Here's how the part is built. I have some questions about the finished solid (model axes, mm). A direction names the side the tool comes from. Round coordinates to 2 decimals unless told otherwise and drop trailing zeros. Order: outer loops, then holes, each group sorted by start corner. A loop starts at its lowest first (then second) coordinate and runs counter-clockwise, first axis right, second up. Notation, with made-up numbers: (-38, 80) -> (8, 80) arc R24 cw to (8, 92) -> close; hole circle Ø6 at (-5.5, 81). An arc over 180 degrees is marked (long way). One line per item, written item: value.
```python
from build123d import *
from build123d.topology import SkipClean

# Parameters (mm, degrees)
SKETCH_2_R          = 4.9
EXTRUDE_1_DEPTH     = 9
EXTRUDE_2_DEPTH     = 10
SKETCH_4_R          = 1.5
CUT_EXTRUDE_1_DEPTH = 22.46392322
SKETCH_5_R          = 3.35
EXTRUDE_3_DEPTH     = 34
CHAMFER_1_SIZE      = 1


with BuildPart() as part:
    # 草图2 → 凸台-拉伸1 (new body)
    with BuildSketch(Plane.XY):
        Circle(SKETCH_2_R)
    extrude(amount=EXTRUDE_1_DEPTH)

    # 草图3 → 凸台-拉伸2 (add)
    with SkipClean():  # the faces are left unmerged after this step: merging them gives an invalid solid
        with BuildSketch(Plane.XY.offset(9)):
            with BuildLine():
                Line((-1.8, -4.557411546), (-1.8, 4.557411546))
                ThreePointArc((-1.8, 4.557411546), (-2.894085134, 3.954019631), (-3.8, 3.09354166))
                Line((-3.8, 3.09354166), (-3.8, -3.09354166))
                ThreePointArc((-3.8, -3.09354166), (-2.894085134, -3.954019631), (-1.8, -4.557411546))
            make_face()
            with BuildLine():
                Line((1.8, -4.557411546), (1.8, 4.557411546))
                ThreePointArc((1.8, 4.557411546), (2.894085134, 3.954019631), (3.8, 3.09354166))
                Line((3.8, 3.09354166), (3.8, -3.09354166))
                ThreePointArc((3.8, -3.09354166), (2.894085134, -3.954019631), (1.8, -4.557411546))
            make_face()
        extrude(amount=EXTRUDE_2_DEPTH)

    # 草图4 → 切除-拉伸1 (cut, through all)
    with SkipClean():  # the faces are left unmerged after this step: merging them gives an invalid solid
        with BuildSketch(Plane.ZY.offset(3.8)):
            with Locations((16.318814586, 0)):
                Circle(SKETCH_4_R)
        extrude(amount=-CUT_EXTRUDE_1_DEPTH, mode=Mode.SUBTRACT)

    # 草图5 → 凸台-拉伸3 (add)
    with SkipClean():  # the faces are left unmerged after this step: merging them gives an invalid solid
        with BuildSketch(Plane(origin=(0, 0, 0), x_dir=(-1, 0, 0), z_dir=(0, 0, -1))):
            with Locations(Location((0, 0, 0), (0, 0, 180))):
                Circle(SKETCH_5_R)
        extrude(amount=EXTRUDE_3_DEPTH)

    # 倒角1
    chamfer_1_edges = [part.edges().sort_by_distance(p)[0] for p in [
        (-3.35, 0, -34),
    ]]
    chamfer(chamfer_1_edges, length=CHAMFER_1_SIZE)


solid = part.part
```
Q1. I want a section at A-A on z = 13. Write out the boundary of the cut face in (x, y), then the cut area to 3 significant figures.
Answers:
outline: (-3.8, -3.09) arc R4.9 ccw to (-1.8, -4.56) -> (-1.8, 4.56) arc R4.9 ccw to (-3.8, 3.09) -> close; (1.8, -4.56) arc R4.9 ccw to (3.8, -3.09) -> (3.8, 3.09) arc R4.9 ccw to (1.8, 4.56) -> close
area: 31.7 mm2
Q2. I want a section at B-B on x = 0. Write out the boundary of the cut face in (y, z), then the cut area to 3 significant figures.
Answers:
outline: (-4.9, 0) -> (-3.35, 0) -> (-3.35, -33) -> (-2.35, -34) -> (2.35, -34) -> (3.35, -33) -> (3.35, 0) -> (4.9, 0) -> (4.9, 9) -> (-4.9, 9) -> close
area: 315 mm2
Q3. Which directions (+Z, -Z, +X, -X, +Y, -Y) give clear straight access to the entire face, cutting with the end or side of a thin tool? Please do faces 5 (the face through (-4, 0, 9)), 6 (the face through (-3, 0, 19)), 7 (the face through (0, 0, 9)), 8 (the face through (4, 0, 9)).
Answers:
face 5: +Z, -X, +Y, -Y
face 6: +Z, +X, -X, +Y, -Y
face 7: +Z, +Y, -Y
face 8: +Z, +X, +Y, -Y
Q4. I want a section at C-C on y = 0. Write out the boundary of the cut face in (x, z).
Answers:
outline: (-4.9, 0) -> (-3.35, 0) -> (-3.35, -33) -> (-2.35, -34) -> (2.35, -34) -> (3.35, -33) -> (3.35, 0) -> (4.9, 0) -> (4.9, 9) -> (3.8, 9) -> (3.8, 14.82) -> (1.8, 14.82) -> (1.8, 9) -> (-1.8, 9) -> (-1.8, 14.82) -> (-3.8, 14.82) -> (-3.8, 9) -> (-4.9, 9) -> close; (-3.8, 17.82) -> (-1.8, 17.82) -> (-1.8, 19) -> (-3.8, 19) -> close; (1.8, 17.82) -> (3.8, 17.82) -> (3.8, 19) -> (1.8, 19) -> close
Q5. If we mould it in two halves opening along Y, with no side actions, what happens to faces 1 (the face through (2, -3, 0)), 2 (the face through (-0.73, 3.27, -16.27)), 3 (the face through (-2.81, 0.07, 14.82)), 4 (the face through (2.79, 0.07, 14.82))? For each: pulls with the +Y half, pulls with the -Y half, needs draft (parallel to the pull), parting line crosses it, or undercut.
Answers:
face 1: needs draft
face 2: parting line crosses it
face 3: undercut
face 4: undercut
Q6. For P1, Ø1.1, axis at x = 0.5, y = 0.5, coming from the +Z side; P2, Ø4.5, axis at y = -0.5, z = 12.5, coming from the +X side; P3, Ø3, axis at x = -2, z = -24, coming from the +Y side, each with a flat end and sliding along its axis, tell me the tip position at first contact or that it passes through.
Answers:
P1: z = 9
P2: x = 3.8
P3: y = 3.31
Q7. I need wall thicknesses on line 1 along X through (y, z) = (-2.5, 10.5); line 2 along X through (y, z) = (0.25, -29.5); line 3 along Z through (x, y) = (-0.75, 0). Which ranges of each line are inside material? Lowest first, please.
Answers:
line 1: -3.8 to -1.8, 1.8 to 3.8
line 2: -3.34 to 3.34
line 3: -34 to 9
Q8. I want a section at D-D on z = -12. Write out the boundary of the cut face in (x, y), then the cut area to 3 significant figures.
Answers:
outline: circle Ø6.7 at (0, 0)
area: 35.3 mm2
